CAD build for the part. Positions are in the model's coordinates, mm. Round coordinates to 2 decimals unless told otherwise and drop trailing zeros. Order: outer loops, then holes, each group sorted by start corner. A loop starts at its lowest first (then second) coordinate and runs counter-clockwise, first axis right, second up. Notation, with made-up numbers: M 23.5,9.25 L 56.5,9.25 A14 ccw 56.5,36.25 Z; hole C 44.25,0 d1. An arc over 180 degrees is marked long. Answer as a JSON object with one key per item and string values.
```python
from build123d import *

# Parameters (mm, degrees)
ESQUISSE1_R             = 1.5
ESQUISSE1_R_2           = 1.499999995
ESQUISSE1_R_3           = 1.500000001
BOSS_EXTRU_1_DEPTH      = 5
ESQUISSE2_R             = 1.5
ENL_V_MAT_EXTRU_1_DEPTH = 5


with BuildPart() as part:
    # Esquisse1 → Boss.-Extru.1 (new body)
    with BuildSketch(Plane(origin=(0, 0, 0), x_dir=(1, 0, 0), z_dir=(0, 1, 0))):
        Polygon((-60, 110), (-60, 160), (60, 160), (60, 110), (110, 110), (110, -110), (60, -110), (60, -160), (-60, -160), (-60, -110), (-110, -110), (-110, 0), (-110, 110), align=None)
        with Locations(Location((-105, -105, 0), (0, 0, 270))):
            Circle(ESQUISSE1_R, mode=Mode.SUBTRACT)
        with Locations(Location((-105, -55, 0), (0, 0, 270))):
            Circle(ESQUISSE1_R, mode=Mode.SUBTRACT)
        with Locations(Location((-55, -105, 0), (0, 0, 270))):
            Circle(ESQUISSE1_R, mode=Mode.SUBTRACT)
        with Locations(Location((-55, -155, 0), (0, 0, 270))):
            Circle(ESQUISSE1_R, mode=Mode.SUBTRACT)
        with Locations(Location((-55, 155, 0), (0, 0, 90))):
            Circle(ESQUISSE1_R, mode=Mode.SUBTRACT)
        with Locations(Location((-55, 105, 0), (0, 0, 90))):
            Circle(ESQUISSE1_R, mode=Mode.SUBTRACT)
        with Locations(Location((-105, 105, 0), (0, 0, 90))):
            Circle(ESQUISSE1_R, mode=Mode.SUBTRACT)
        with Locations(Location((-105, 55, 0), (0, 0, 90))):
            Circle(ESQUISSE1_R, mode=Mode.SUBTRACT)
        with Locations(Location((55, -155, 0), (0, 0, 90))):
            Circle(ESQUISSE1_R, mode=Mode.SUBTRACT)
        with Locations(Location((55, -105, 0), (0, 0, 90))):
            Circle(ESQUISSE1_R, mode=Mode.SUBTRACT)
        with Locations(Location((105, -105, 0), (0, 0, 90))):
            Circle(ESQUISSE1_R, mode=Mode.SUBTRACT)
        with Locations(Location((105, 105, 0), (0, 0, 270))):
            Circle(ESQUISSE1_R, mode=Mode.SUBTRACT)
        with Locations(Location((55, 105, 0), (0, 0, 270))):
            Circle(ESQUISSE1_R, mode=Mode.SUBTRACT)
        with Locations(Location((55, 155, 0), (0, 0, 270))):
            Circle(ESQUISSE1_R, mode=Mode.SUBTRACT)
        with Locations(Location((-20.263921607, -83.580815365, 0), (0, 0, 270))):
            Circle(ESQUISSE1_R, mode=Mode.SUBTRACT)
        with Locations(Location((20.686866729, -83.580815365, 0), (0, 0, 270))):
            Circle(ESQUISSE1_R_2, mode=Mode.SUBTRACT)
        with Locations(Location((22.476974657, -127.410006662, 0), (0, 0, 270))):
            Circle(ESQUISSE1_R_3, mode=Mode.SUBTRACT)
        with Locations(Location((-21.804614529, -127.50597342, 0), (0, 0, 270))):
            Circle(ESQUISSE1_R, mode=Mode.SUBTRACT)
        Polygon((-40, 138.836374596), (40, 138.836374596), (40, 87), (87, 87), (87, -87), (31.326862642, -87), (31.326862642, -73.839408228), (-31.326862646, -73.839408228), (-31.326862646, -87), (-87, -87), (-87, 87), (-40, 87), align=None, mode=Mode.SUBTRACT)
        with BuildLine():
            add(Edge.make_bspline(
                [(0.293780888, -76.726336566), (-0.996088195, -76.578291907), (-4.699230167, -77.207421086), (-11.368955783, -80.020833344), (-17.338132033, -84.895696313), (-23.699116857, -93.09913388), (-26.473794847, -103.394022574), (-26.398842017, -120.164373886), (-18.920830658, -125.430457585), (-12.734895056, -130.805440699), (-5.32063418, -133.167404841), (-1.132230329, -133.810542206), (0.293780888, -133.661970747)],
                knots=[0, 0, 0, 0, 0.044371954, 0.129133426, 0.24755985, 0.307901827, 0.482602167, 0.644889464, 0.731533462, 0.853727, 0.909620458, 1, 1, 1, 1], degree=3))
            add(Edge.make_bspline(
                [(0.293780888, -76.726336566), (1.583649972, -76.578291907), (5.286791943, -77.207421086), (11.95651756, -80.020833344), (17.925693809, -84.895696313), (24.286678634, -93.09913388), (27.061356623, -103.394022574), (26.986403794, -120.164373886), (19.508392434, -125.430457585), (13.322456832, -130.805440699), (5.908195957, -133.167404841), (1.719792105, -133.810542206), (0.293780888, -133.661970747)],
                knots=[0, 0, 0, 0, 0.044371954, 0.129133426, 0.24755985, 0.307901827, 0.482602167, 0.644889464, 0.731533462, 0.853727, 0.909620458, 1, 1, 1, 1], degree=3))
        make_face(mode=Mode.SUBTRACT)
    extrude(amount=BOSS_EXTRU_1_DEPTH)

    # Esquisse2 → Enlèv. mat.-Extru.1 (cut)
    with BuildSketch(Plane(origin=(0, 5, 0), x_dir=(1, 0, 0), z_dir=(0, 1, 0))):
        with Locations(Location((-105, -80, 0), (0, 0, 270))):
            Circle(ESQUISSE2_R)
        with Locations(Location((-80, -105, 0), (0, 0, 270))):
            Circle(ESQUISSE2_R)
        with Locations(Location((-55, -130, 0), (0, 0, 270))):
            Circle(ESQUISSE2_R)
        with Locations(Location((55, -130, 0), (0, 0, 270))):
            Circle(ESQUISSE2_R)
        with Locations(Location((80, -105, 0), (0, 0, 270))):
            Circle(ESQUISSE2_R)
        with Locations(Location((105, -80, 0), (0, 0, 270))):
            Circle(ESQUISSE2_R)
        with Locations(Location((105, 80, 0), (0, 0, 270))):
            Circle(ESQUISSE2_R)
        with Locations(Location((80, 105, 0), (0, 0, 270))):
            Circle(ESQUISSE2_R)
        with Locations(Location((55, 130, 0), (0, 0, 270))):
            Circle(ESQUISSE2_R)
        with Locations(Location((-55, 130, 0), (0, 0, 270))):
            Circle(ESQUISSE2_R)
        with Locations(Location((-80, 105, 0), (0, 0, 270))):
            Circle(ESQUISSE2_R)
        with Locations(Location((-105, 80, 0), (0, 0, 270))):
            Circle(ESQUISSE2_R)
    extrude(amount=-ENL_V_MAT_EXTRU_1_DEPTH, mode=Mode.SUBTRACT)


solid = part.part
```
Item 1: Drop a flat-ended pin along its axis: pin 1 Ø3 at (x, y) = (-86.5, 3.5) entering from +Z. Give the stop position or say it passes through.
Worked answers:
{"pin 1": "stops at z = 110"}
Item 2: Saw through at A-A on z = -92. List the corners of the cut face in (x, y), and give its area (3 significant figures).
Worked answers:
{"outline": "M -110,0 L -40,0 L -40,5 L -110,5 Z; M 40,0 L 110,0 L 110,5 L 40,5 Z", "area": "700 mm2"}
Item 3: Wall check: line 1 along X through (y, z) = (0.75, 74); line 2 along Z through (x, y) = (105, 3); line 3 along Z through (x, y) = (28, 1.5). Give the ranges that are in metal, low to high. Write a range as [from, to].
Worked answers:
{"line 1": "x = [-110, -87], [-31.33, 31.33], [87, 110]", "line 2": "z = [-110, -106.5], [-103.5, -81.5], [-78.5, 78.5], [81.5, 103.5], [106.5, 110]", "line 3": "z = [-160, -138.84], [73.84, 160]"}
Item 4: Saw through at B-B on x = -9. State how many separate pieces and enclosed holes the cut face has, and give its area (3 significant figures).
Worked answers:
{"separate pieces": "3", "enclosed holes": "0", "area": "273 mm2"}
